Design review of the part built by this model. Coordinates are the model's own, in mm. Round coordinates to 2 decimals unless told otherwise and drop trailing zeros. Order: outer loops, then holes, each group sorted by start corner. A loop starts at its lowest first (then second) coordinate and runs counter-clockwise, first axis right, second up. Notation, with made-up numbers: (61, 86.5) - (94, 86.5) arc R34 cw to (94, 125.5) - close; hole circle Ø11 at (-36, -9). An arc over 180 degrees is marked (long way). Write item = value, one per line.
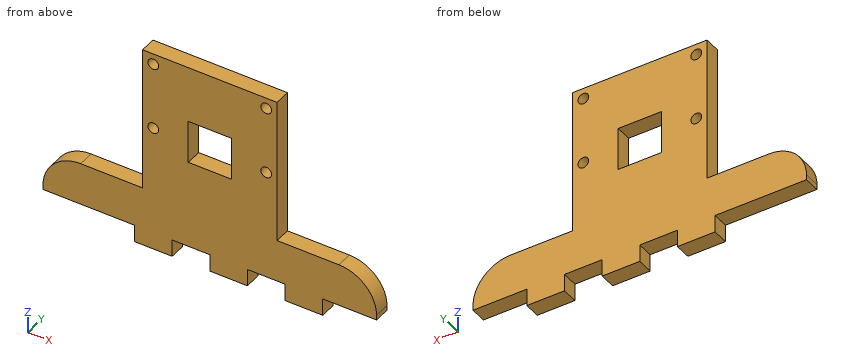
from build123d import *

# Parameters (mm, degrees)
F0_R     = 1
F0_W     = 8
F0_H     = 8
F1_DEPTH = 1.5


with BuildPart() as f1:
    # F0 (on Front) → F1 (new body, symmetric)
    with BuildSketch(Plane.XZ):
        with BuildLine():
            Line((12.5, -13.5), (12.5, 13.5))
            Line((12.5, 13.5), (-12.5, 13.5))
            Line((-12.5, 13.5), (-12.5, -13.5))
            Line((-12.5, -13.5), (-24, -13.5))
            ThreePointArc((-24, -13.5), (-28.949747, -15.550253), (-31, -20.5))
            Line((-31, -20.5), (-31, -21.411933))
            Line((-31, -21.411933), (-14, -21.411933))
            Line((-14, -21.411933), (-14, -24.611933))
            Line((-14, -24.611933), (-7, -24.611933))
            Line((-7, -24.611933), (-7, -21.411933))
            Line((-7, -21.411933), (0, -21.411933))
            Line((0, -21.411933), (0, -24.611933))
            Line((0, -24.611933), (7, -24.611933))
            Line((7, -24.611933), (7, -21.411933))
            Line((7, -21.411933), (14, -21.411933))
            Line((14, -21.411933), (14, -24.611933))
            Line((14, -24.611933), (21, -24.611933))
            Line((21, -24.611933), (21, -21.411113))
            Line((21, -21.411113), (31, -21.411378))
            Line((31, -21.411378), (31, -20.5))
            ThreePointArc((31, -20.5), (28.949747, -15.550253), (24, -13.5))
            Line((24, -13.5), (12.5, -13.5))
        make_face()
        with Locations((-10.5, -1)):
            Circle(F0_R, mode=Mode.SUBTRACT)
        with Locations((-10.5, 11.5)):
            Circle(F0_R, mode=Mode.SUBTRACT)
        with Locations((0, -1)):
            Rectangle(F0_W, F0_H, mode=Mode.SUBTRACT)
        with Locations((10.5, -1)):
            Circle(F0_R, mode=Mode.SUBTRACT)
        with Locations((10.5, 11.5)):
            Circle(F0_R, mode=Mode.SUBTRACT)
    extrude(amount=F1_DEPTH, both=True)


solid = f1.part
Item 1: For line 1 along Z through (x, y) = (-10.5, 0.1); line 2 along Z through (x, y) = (10.5, 0.55); line 3 along Z through (x, y) = (-21, -0.85), list the stretches that pass through material, from the lowest coordinate up. Write a range as [from, to].
Data:
line_1 = [-24.61, -2], [0, 10.5], [12.5, 13.5]
line_2 = [-21.41, -2], [0, 10.5], [12.5, 13.5]
line_3 = [-21.41, -13.5]
Item 2: Take a section at D-D, the plane y = 0. Count the separate pieces of the cut face and the enclosed holes in it, and give its area (3 significant figures).
Data:
separate_pieces = 1
enclosed_holes = 5
area = 1,140 mm2
Item 3: Insertion check: P1, Ø0.9, axis at x = 27, y = 0.5, coming from the -Z side; P2, Ø1.5, axis at y = -0.5, z = -4.5, coming from the -X side; P3, Ø1.5, axis at y = 0, z = -22.5, coming from the -X side. Each pin has a flat end and moves straight along its axis. Give the tip position at first contact, or say it passes through.
Data:
P1 = -21.41
P2 = -12.5
P3 = -14
Item 4: Take a section at A-A, the plane x = -10.5. State the section outline as (y, z) points, and give its area (3 significant figures).
Data:
outline = (-1.5, -24.61) - (1.5, -24.61) - (1.5, -2) - (-1.5, -2) - close; (-1.5, 0) - (1.5, 0) - (1.5, 10.5) - (-1.5, 10.5) - close; (-1.5, 12.5) - (1.5, 12.5) - (1.5, 13.5) - (-1.5, 13.5) - close
area = 102 mm2
Item 5: Take a section at B-B, the plane z = 11.5. State the section outline as (x, y) points, and give its area (3 significant figures).
Data:
outline = (-12.5, -1.5) - (-11.5, -1.5) - (-11.5, 1.5) - (-12.5, 1.5) - close; (-9.5, -1.5) - (9.5, -1.5) - (9.5, 1.5) - (-9.5, 1.5) - close; (11.5, -1.5) - (12.5, -1.5) - (12.5, 1.5) - (11.5, 1.5) - close
area = 63.0 mm2
Item 6: Take a section at C-C, the plane z = -1. State the section outline as (x, y) points, and give its area (3 significant figures).
Data:
outline = (-12.5, -1.5) - (-11.5, -1.5) - (-11.5, 1.5) - (-12.5, 1.5) - close; (-9.5, -1.5) - (-4, -1.5) - (-4, 1.5) - (-9.5, 1.5) - close; (4, -1.5) - (9.5, -1.5) - (9.5, 1.5) - (4, 1.5) - close; (11.5, -1.5) - (12.5, -1.5) - (12.5, 1.5) - (11.5, 1.5) - close
area = 39.0 mm2
